```python
from build123d import *

# Parameters (mm, degrees)
SKETCH1_R           = 18
BOSS_EXTRUDE1_DEPTH = 62
SKETCH2_R           = 6.7
BOSS_EXTRUDE2_DEPTH = 4.68
SKETCH3_R           = 1.585
BOSS_EXTRUDE3_DEPTH = 13.6
SKETCH4_R           = 1.8
CUT_EXTRUDE1_DEPTH  = 20


with BuildPart() as part:
    # Sketch1 → Boss-Extrude1 (new body)
    with BuildSketch(Plane(origin=(0, 0, 0), x_dir=(0, 0, -1), z_dir=(1, 0, 0))):
        Circle(SKETCH1_R)
    extrude(amount=BOSS_EXTRUDE1_DEPTH)

    # Sketch2 → Boss-Extrude2 (add)
    with BuildSketch(Plane(origin=(62, 0, 0), x_dir=(0, 0, -1), z_dir=(1, 0, 0))):
        with Locations(Location((0, 0, 0), (0, 0, 180))):
            Circle(SKETCH2_R)
    extrude(amount=BOSS_EXTRUDE2_DEPTH)

    # Sketch3 → Boss-Extrude3 (add)
    with BuildSketch(Plane(origin=(66.68, 0, 0), x_dir=(0, 0, -1), z_dir=(1, 0, 0))):
        Circle(SKETCH3_R)
    extrude(amount=BOSS_EXTRUDE3_DEPTH)

    # Sketch4 → Cut-Extrude1 (cut)
    with BuildSketch(Plane(origin=(62, 0, 0), x_dir=(0, 0, -1), z_dir=(1, 0, 0))):
        with Locations((-12.565, 0)):
            Circle(SKETCH4_R)
        with Locations((12.565, 0)):
            Circle(SKETCH4_R)
    extrude(amount=-CUT_EXTRUDE1_DEPTH, mode=Mode.SUBTRACT)


solid = part.part
```
Geometry: final body of the model. Coordinates: model frame, mm. A direction names the side the tool comes from. Coordinates: 2 decimals unless noted, no trailing zeros. Order: outer loops, then holes, each group sorted by start corner. A loop starts at its lowest first (then second) coordinate and runs counter-clockwise, first axis right, second up. Notation, with made-up numbers: (52, -31) -> (96, -31) arc R22 cw to (96, -17) -> close; hole circle Ø2 at (41.5, 3). An arc over 180 degrees is marked (long way). Use CSV: the item, a comma, the result in double quotes.
1) Mould query, pull axis Y, two halves, no side actions, for faces 1 (the cylindrical face through (64.31, 6.54, -1.45)), 2 (the flat face through (62, -8, 0)), 3 (the flat face through (42, 0, 13)). Classes: +Y half, -Y half, draft (parallel to the pull), parting line (faces both ways), or undercut.
Findings:
face 1,"parting line"
face 2,"draft"
face 3,"undercut"
2) Section D-D on z = 8.5. Output: boundary loops of the cut face in (x, y).
Findings:
outline,"(0, -15.87) -> (62, -15.87) -> (62, 15.87) -> (0, 15.87) -> close"
3) Section A-A on z = 0. Output: boundary loops of the cut face in (x, y) (3 decimals), then the cut area to 3 significant figures.
Findings:
outline,"(0, -18) -> (62, -18) -> (62, -6.7) -> (66.68, -6.7) -> (66.68, -1.585) -> (80.28, -1.585) -> (80.28, 1.585) -> (66.68, 1.585) -> (66.68, 6.7) -> (62, 6.7) -> (62, 18) -> (0, 18) -> close"
area,"2,340 mm^2"
4) Line query: line 1 (X direction, y = 8.5, z = -3); line 2 (X direction, y = -3, z = 0.5); line 3 (Y direction, x = 29.5, z = 5). Output: solid intervals per line, ascending.
Findings:
line 1,"x = 0 to 62"
line 2,"x = 0 to 66.68"
line 3,"y = -17.29 to 17.29"
5) Section B-B on y = 0. Output: boundary loops of the cut face in (x, z) (3 decimals), then the cut area to 3 significant figures.
Findings:
outline,"(0, -18) -> (62, -18) -> (62, -14.365) -> (42, -14.365) -> (42, -10.765) -> (62, -10.765) -> (62, -6.7) -> (66.68, -6.7) -> (66.68, -1.585) -> (80.28, -1.585) -> (80.28, 1.585) -> (66.68, 1.585) -> (66.68, 6.7) -> (62, 6.7) -> (62, 10.765) -> (42, 10.765) -> (42, 14.365) -> (62, 14.365) -> (62, 18) -> (0, 18) -> close"
area,"2,190 mm^2"
6) Access query for faces 4 (the flat face through (42, 0, -13)), 5 (the flat face through (80.28, 0, 0)). Directions: +Z, -Z, +X, -X, +Y, -Y. A direction counts if a zero-diameter tool reaches every point of the face in a straight line with its end or side. Return the directions, or none.
Findings:
face 4,"+X"
face 5,"+Z, -Z, +X, +Y, -Y"
7) Pin query (flat end, axial travel): pin 1 Ø3 at (y, z) = (0, -12.565) entering from +X; pin 2 Ø1 at (x, z) = (25.5, 1.5) entering from -Y; pin 3 Ø1 at (x, z) = (28, -8) entering from +Y. Return the tip coordinate at first contact, or that it passes through.
Findings:
pin 1,"stops at x = 42"
pin 2,"stops at y = -17.97"
pin 3,"stops at y = 16.36"
8) Section C-C on x = 30.5. Output: boundary loops of the cut face in (y, z).
Findings:
outline,"circle Ø36 at (0, 0)"
